Answer from the drawing. Dimensions are ordinates in mm from the lowest x, y and z of the part. A direction names the side the tool comes from. Coordinates: 2 decimals unless noted, no trailing zeros. Write each loop counter-clockwise with the first axis right and the second up, starting at its lowest first coordinate (ties: lowest second). Pieces come first, ordered by that corner, then holes. Notation, with made-up numbers: (9.5, 60.25) - (48.5, 60.25) arc R36 cw to (48.5, 96.25) - close; hole circle Ø7 at (-15.75, 2). An arc over 180 degrees is marked (long way). Use a Markdown table: item, result.
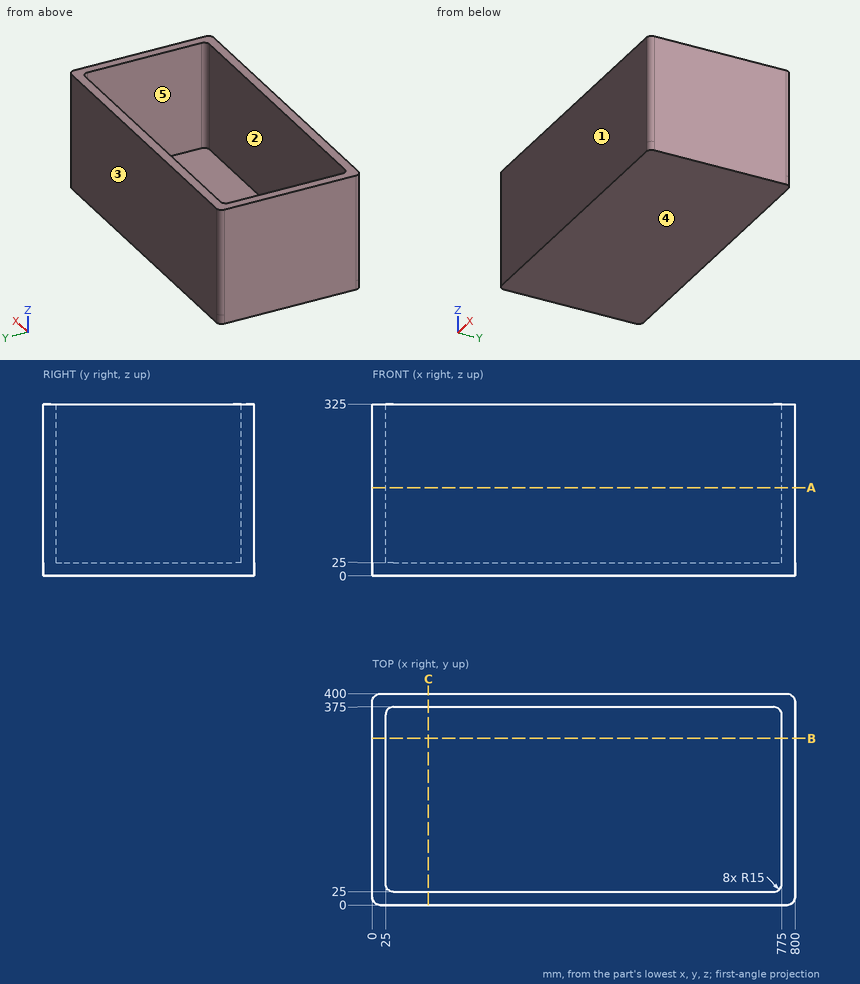
(1) A cutting plane is placed at A-A, the plane z = 166.5. Write down the section's boundary in (x, y), and give its area (3 significant figures).
Report:
| item | result |
|---|---|
| outline | (0, 15) arc R15 ccw to (15, 0) - (785, 0) arc R15 ccw to (800, 15) - (800, 385) arc R15 ccw to (785, 400) - (15, 400) arc R15 ccw to (0, 385) - close; hole (25, 40) arc R15 ccw to (40, 25) - (760, 25) arc R15 ccw to (775, 40) - (775, 360) arc R15 ccw to (760, 375) - (40, 375) arc R15 ccw to (25, 360) - close |
| area | 57,500 mm² |
(2) A cutting plane is placed at C-C, the plane x = 106. Write down the section's boundary in (y, z), and give its area (3 significant figures).
Report:
| item | result |
|---|---|
| outline | (0, 0) - (400, 0) - (400, 325) - (375, 325) - (375, 25) - (25, 25) - (25, 325) - (0, 325) - close |
| area | 25,000 mm² |
(3) A cutting plane is placed at B-B, the plane y = 315.5. Write down the section's boundary in (x, z), and give its area (3 significant figures).
Report:
| item | result |
|---|---|
| outline | (0, 0) - (800, 0) - (800, 325) - (775, 325) - (775, 25) - (25, 25) - (25, 325) - (0, 325) - close |
| area | 35,000 mm² |
(4) Straight lines are drawn through the part: L1, parallel to X at y = 317, z = 157; L2, parallel to Y at x = 603.5, z = 165; L3, parallel to Z at x = 40.5, y = 279.5. For each, find the intervals that lie inside material, in ascending order.
Report:
| item | result |
|---|---|
| L1 | x = 0 to 25, 775 to 800 |
| L2 | y = 0 to 25, 375 to 400 |
| L3 | z = 0 to 25 |
(5) Each of these flat-tipped pins is pushed along its axis until it touches: P1, Ø2, axis at x = 476, y = 180, coming from the +Z side; P2, Ø2, axis at x = 527.5, y = 271, coming from the -Z side. Where does it stop, or does it pass through?
Report:
| item | result |
|---|---|
| P1 | stops at z = 25 |
| P2 | stops at z = 0 |
(6) The mould has two halves that part along Y. Classify the marked faces 1, 2 and 3: pulls with the +Y half, pulls with the -Y half, needs draft (parallel to the pull), parting line crosses it, or undercut.
Report:
| item | result |
|---|---|
| face 1 | pulls with the -Y half |
| face 2 | undercut |
| face 3 | pulls with the +Y half |
(7) For the marked faces 4 and 5, determine the directions among +Z, -Z, +X, -X, +Y, -Y from which every point of the face is accessible in a straight line to the end or side of a thin tool.
Report:
| item | result |
|---|---|
| face 4 | -Z, +X, -X, +Y, -Y |
| face 5 | +Z |
